from build123d import *

# Parameters (mm, degrees)
SKETCH1_W            = 600
SKETCH1_H            = 450
BOSS_EXTRUDE1_DEPTH  = 30
FILLET1_R            = 30
SKETCH2_W            = 347.887186226
SKETCH2_H            = 352.796759622
BOSS_EXTRUDE2_DEPTH  = 80
RIB2_REACH           = 385.438
SKETCH3_WALL_W       = 918.175870934
SKETCH3_WALL_H       = 100
SKETCH4_R            = 35
BOSS_EXTRUDE3_DEPTH  = 300
BOSS_EXTRUDE4_DEPTH  = 60
BOSS_EXTRUDE5_DEPTH  = 18
MIRROR3_COPY_1_DEPTH = 18


with BuildPart() as part:
    # Sketch1 → Boss-Extrude1 (new body)
    with BuildSketch(Plane.XY):
        Rectangle(SKETCH1_W, SKETCH1_H)
    extrude(amount=BOSS_EXTRUDE1_DEPTH)

    # Fillet1
    fillet1_edges = [part.edges().sort_by_distance(p)[0] for p in [
        (300, -225, 15),
        (-300, -225, 15),
        (-300, 225, 15),
        (300, 225, 15),
    ]]
    fillet(fillet1_edges, radius=FILLET1_R)

    # Sketch2 → Boss-Extrude2 (add)
    with BuildSketch(Plane(origin=(0, 0, 0), x_dir=(-1, 0, 0), z_dir=(0, 0, -1))):
        Rectangle(SKETCH2_W, SKETCH2_H)
    extrude(amount=BOSS_EXTRUDE2_DEPTH)

    # Sketch3 wall → Rib2 (add, up to next)
    with BuildSketch(Plane(origin=(236.971796557, 0, -40), x_dir=(0.844321344916, 0, 0.535837164182), z_dir=(0.535837164182, 0, -0.844321344916)), mode=Mode.PRIVATE) as rib2_sk1:
        Rectangle(SKETCH3_WALL_W, SKETCH3_WALL_H)
    rib2_tool1 = extrude(rib2_sk1.sketch, amount=-RIB2_REACH, mode=Mode.PRIVATE) - part.part
    rib2 = rib2_tool1.solids().sort_by_distance((236.971796557, 0, -40))[0]
    add(rib2)

    # Mirror1: Rib2 across plane
    add(rib2.mirror(Plane(origin=(0, 0, 0), x_dir=(0, 0, 1), z_dir=(1, 0, 0))))

    # Sketch4 → Boss-Extrude3 (add)
    with BuildSketch(Plane.XY.offset(30)):
        with Locations((-70, 0)):
            Circle(SKETCH4_R)
        with Locations((70, 0)):
            Circle(SKETCH4_R)
    extrude(amount=BOSS_EXTRUDE3_DEPTH)

    # Sketch5 → Boss-Extrude4 (add)
    with BuildSketch(Plane(origin=(0, 0, -80), x_dir=(-1, 0, 0), z_dir=(0, 0, -1))):
        Polygon((86.602540378, 0), (43.301270189, 75), (-43.301270189, 75), (-86.602540378, 0), (-43.301270189, -75), (43.301270189, -75), align=None)
    extrude(amount=BOSS_EXTRUDE4_DEPTH)

    # Sketch6 → Boss-Extrude5 (add)
    with BuildSketch(Plane(origin=(0, 0, 0), x_dir=(-1, 0, 0), z_dir=(0, 0, -1))):
        Polygon((-230.886428661, 176.398379811), (-242.973945963, 197.334573917), (-267.148980569, 197.334573917), (-279.236497871, 176.398379811), (-267.148980569, 155.462185706), (-242.973945963, 155.462185706), align=None)
    boss_extrude5 = extrude(amount=BOSS_EXTRUDE5_DEPTH)

    # Mirror2: Boss-Extrude5 across plane
    add(boss_extrude5.mirror(Plane(origin=(0, 0, 0), x_dir=(0, 0, 1), z_dir=(1, 0, 0))))

    # Mirror3: Boss-Extrude5 across plane
    add(boss_extrude5.mirror(Plane.ZX))

    # Mirror3 copy 1 sketch → Mirror3 copy 1 (add)
    with BuildSketch(Plane(origin=(0, 0, 0), x_dir=(1, 0, 0), z_dir=(0, 0, -1))):
        Polygon((-230.886428661, 176.398379811), (-242.973945963, 197.334573917), (-267.148980569, 197.334573917), (-279.236497871, 176.398379811), (-267.148980569, 155.462185706), (-242.973945963, 155.462185706), align=None)
    extrude(amount=MIRROR3_COPY_1_DEPTH)


solid = part.part
Input: part model. Units: mm. Frame: model coordinates. A direction names the side the tool comes from. Coordinates: 2 decimals unless noted, no trailing zeros. Loops run counter-clockwise (first coordinate to the right, second up) from the corner with the lowest first, then second, coordinate; pieces in that order, holes last. Notation, with made-up numbers: (-3, 37.5) - (34, 37.5) arc R36 cw to (34, 72.5) - close; hole circle Ø6 at (-13, 54). An arc over 180 degrees is marked (long way). Answer in a Markdown table with one row per item. Add a question column.
Item 1: Mould query, pull axis Y, two halves, no side actions, for faces 4 (the flat face through (-273.28, -166.08, -8.87)), 5 (the flat face through (-4, 225, 15)), 6 (the flat face through (237.015, -165.784, -8.874)), 7 (the flat face through (1, -75, -110)). Classes: released by +Y, released by -Y, zero draft, split by the parting line, or undercut.
Item 2: Access query for faces 1 (the flat face through (2, 176.398, -39)), 2 (the flat face through (255, 177, -18)), 3 (the flat face through (-273.11, -187.01, -8.87)). Directions: +Z, -Z, +X, -X, +Y, -Y. A direction counts if a zero-diameter tool reaches every point of the face in a straight line with its end or side. Return the directions, or none.
Item 3: Section query A-A on z = 290. Return the cut outline in (x, y), then the cut area to 3 significant figures.
Item 4: Section query B-B on y = 83. Return the cut outline in (x, z), then the cut area to 3 significant figures.
Item 5: Section query D-D on x = -200.5. Return the cut outline in (y, z).
Item 6: Section query C-C on x = 70. Return the cut outline in (y, z).
Item 7: Line query: line 1 along Z through (x, y) = (248, -140.5); line 2 along Y through (x, z) = (72, -50.5); line 3 along X through (y, z) = (26, 214.5). Output: solid intervals per line, ascending. Write a range as [from, to].
Item 8: Contact query for flat-ended pins moving along their axis: P1, Ø20, axis at x = 258.5, z = -11.5, coming from the -Y side; P2, Ø21, axis at x = 258, y = -178.5, coming from the -Z side; P3, Ø12, axis at x = 197, y = 173.5, coming from the -Z side. Output: stop coordinate, or through.
Recorded:
| question | item | result |
|---|---|---|
| 1 | face 4 | undercut |
| 1 | face 5 | released by +Y |
| 1 | face 6 | undercut |
| 1 | face 7 | released by -Y |
| 2 | face 1 | -Z, +Y |
| 2 | face 2 | -Z, +X, +Y |
| 2 | face 3 | -Z, -X, -Y |
| 3 | outline | circle Ø70 at (-70, 0); circle Ø70 at (70, 0) |
| 3 | area | 7,700 mm^2 |
| 4 | outline | (-300, 0) - (-173.94, 0) - (-173.94, -80) - (173.94, -80) - (173.94, 0) - (300, 0) - (300, 30) - (-300, 30) - close |
| 4 | area | 45,800 mm^2 |
| 5 | outline | (-225, 0) - (-50, 0) - (-50, -63.15) - (50, -63.15) - (50, 0) - (225, 0) - (225, 30) - (-225, 30) - close |
| 6 | outline | (-225, 0) - (-176.4, 0) - (-176.4, -80) - (-28.76, -80) - (-28.76, -140) - (28.76, -140) - (28.76, -80) - (176.4, -80) - (176.4, 0) - (225, 0) - (225, 30) - (35, 30) - (35, 330) - (-35, 330) - (-35, 30) - (-225, 30) - close |
| 7 | line 1 | [0, 30] |
| 7 | line 2 | [-176.4, 176.4] |
| 7 | line 3 | [-93.43, -46.57], [46.57, 93.43] |
| 8 | P1 | y = -197.33 |
| 8 | P2 | z = -18 |
| 8 | P3 | z = 0 |
